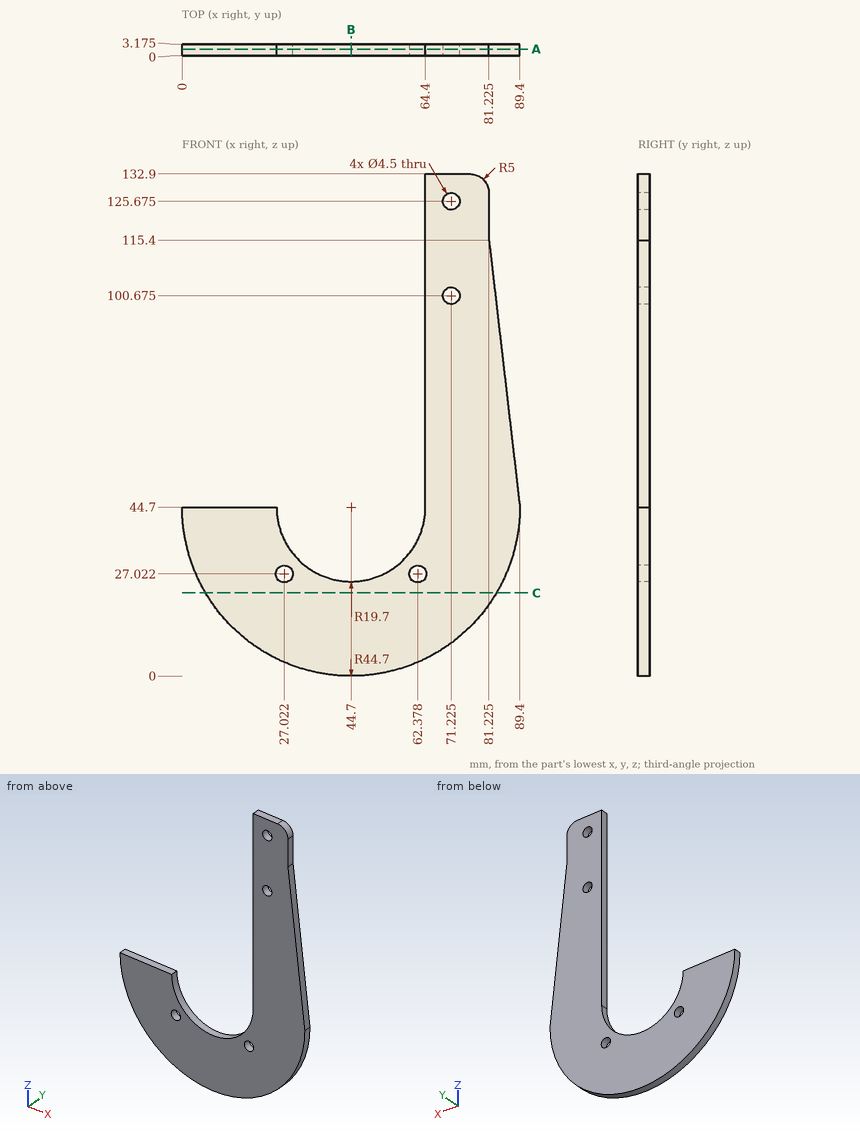
For this review, use the dimensioned drawing (mm, ordinates from the lowest corner) and the shaded views. Coordinates: 2 decimals unless noted, no trailing zeros. Loops run counter-clockwise (first coordinate to the right, second up) from the corner with the lowest first, then second, coordinate; pieces in that order, holes last. Notation, with made-up numbers: (19.5, -9) -> (70.5, -9) arc R26 cw to (70.5, 24) -> close; hole circle Ø11 at (-10, 1.5). An arc over 180 degrees is marked (long way). Use a Markdown table: item, result. Add a question column.
1. Add section B-B on x = 44.7. Write out the cut boundary in (y, z) (1 decimal).
2. Add section C-C on z = 22. Write out the cut boundary in (x, y) (1 decimal).
3. Clearance check with flat-ended pins moving along their axes: pin 1 Ø1.6 at (y, z) = (2.5, 120.5) entering from +X (3 decimals); pin 2 Ø1 at (y, z) = (1.5, 83.5) entering from -X; pin 3 Ø7 at (x, z) = (71.225, 125.675) entering from -Y; pin 4 Ø1.5 at (x, y) = (9.5, 2.5) entering from -Z. State where each tip first meets the part, or that it passes through.
4. To check wall thickness, follow line 1 (X direction, y = 0.95, z = 30) (1 decimal); line 2 (X direction, y = 2.6, z = 122.5) (1 decimal); line 3 (X direction, y = 2.5, z = 36) (1 decimal). State the ranges of each line that lie inside material, in increasing order.
5. Add section A-A on y = 1.8. Give the number of separate pieces and of enclosed holes in the cut face, plus the area to 3 significant figures.
Returned:
| question | item | result |
|---|---|---|
| 1 | outline | (0, 0) -> (3.2, 0) -> (3.2, 25) -> (0, 25) -> close |
| 2 | outline | (6.2, 0) -> (83.2, 0) -> (83.2, 3.2) -> (6.2, 3.2) -> close |
| 3 | pin 1 | stops at x = 81.225 |
| 3 | pin 2 | stops at x = 64.4 |
| 3 | pin 3 | stops at y = 0 |
| 3 | pin 4 | stops at z = 16.22 |
| 4 | line 1 | x = 2.5 to 31.6, 57.8 to 86.9 |
| 4 | line 2 | x = 64.4 to 81.2 |
| 4 | line 3 | x = 0.9 to 27, 62.4 to 88.5 |
| 5 | separate pieces | 1 |
| 5 | enclosed holes | 4 |
| 5 | area | 4,230 mm² |
